```python
from build123d import *

# Parameters (mm, degrees)
BASE_DEPTH          = 3
SKETCH2_R           = 1.5
CUT_EXTRUDE1_DEPTH  = 37.373066959
CUT_EXTRUDE2_DEPTH  = 37.373066959
SKETCH6_R           = 3
CUT_EXTRUDE3_DEPTH  = 1.5
CHAMFER2_SIZE       = 0.5
BOSS_EXTRUDE1_START = -2.5
BOSS_EXTRUDE1_DEPTH = 2.5
CUT_EXTRUDE4_START  = -2.5
CUT_EXTRUDE4_DEPTH  = 2.5


# Read off the part's stored shape, not the designer's step: Cut-Extrude4
with BuildPart() as part:
    # Sketch1 → Base (new body)
    with BuildSketch(Plane.XY):
        with BuildLine():
            Line((11, -33), (-11, -33))
            ThreePointArc((-11, -33), (-13.828427125, -31.828427125), (-15, -29))
            Line((-15, -29), (-15, 29))
            ThreePointArc((-15, 29), (-13.828427125, 31.828427125), (-11, 33))
            Line((-11, 33), (11, 33))
            ThreePointArc((11, 33), (13.828427125, 31.828427125), (15, 29))
            Line((15, 29), (15, -29))
            ThreePointArc((15, -29), (13.828427125, -31.828427125), (11, -33))
        make_face()
    extrude(amount=BASE_DEPTH)

    # Sketch2 → Cut-Extrude1 (cut, through all)
    with BuildSketch(Plane.XY.offset(3)):
        with Locations((-11, 29)):
            Circle(SKETCH2_R)
        with Locations((-11, -29)):
            Circle(SKETCH2_R)
        with Locations((11, -29)):
            Circle(SKETCH2_R)
        with Locations((11, 29)):
            Circle(SKETCH2_R)
    extrude(amount=-CUT_EXTRUDE1_DEPTH, mode=Mode.SUBTRACT)

    # Sketch3 → Cut-Extrude2 (cut, through all)
    with BuildSketch(Plane.XY.offset(3)):
        with BuildLine():
            Line((6.5, 29), (6.5, 31))
            Line((6.5, 31), (-6.5, 31))
            Line((-6.5, 31), (-6.5, 29))
            ThreePointArc((-6.5, 29), (-7.818019485, 25.818019485), (-11, 24.5))
            Line((-11, 24.5), (-13, 24.5))
            Line((-13, 24.5), (-13, -24.5))
            Line((-13, -24.5), (-11, -24.5))
            ThreePointArc((-11, -24.5), (-7.818019485, -25.818019485), (-6.5, -29))
            Line((-6.5, -29), (-6.5, -31))
            Line((-6.5, -31), (6.5, -31))
            Line((6.5, -31), (6.5, -29))
            ThreePointArc((6.5, -29), (7.818019485, -25.818019485), (11, -24.5))
            Line((11, -24.5), (13, -24.5))
            Line((13, -24.5), (13, 24.5))
            Line((13, 24.5), (11, 24.5))
            ThreePointArc((11, 24.5), (7.818019485, 25.818019485), (6.5, 29))
        make_face()
    extrude(amount=-CUT_EXTRUDE2_DEPTH, mode=Mode.SUBTRACT)

    # Sketch6 → Cut-Extrude3 (cut)
    with BuildSketch(Plane.XY.offset(3)):
        with Locations((-11, -29)):
            Circle(SKETCH6_R)
        with Locations((11, -29)):
            Circle(SKETCH6_R)
        with Locations((11, 29)):
            Circle(SKETCH6_R)
        with Locations((-11, 29)):
            Circle(SKETCH6_R)
    extrude(amount=-CUT_EXTRUDE3_DEPTH, mode=Mode.SUBTRACT)

    # Chamfer2
    chamfer2_edges = [part.edges().sort_by_distance(p)[0] for p in [
        (7.818019485, 25.818019485, 3),
        (13, 0, 3),
        (7.818019485, -25.818019485, 3),
        (-7.818019485, -25.818019485, 3),
        (-13, 0, 3),
        (-7.818019485, 25.818019485, 3),
        (0, -33, 3),
        (-13.828427125, -31.828427125, 3),
        (-15, 0, 3),
        (-13.828427125, 31.828427125, 3),
        (0, 33, 3),
        (13.828427125, 31.828427125, 3),
        (15, 0, 3),
        (13.828427125, -31.828427125, 3),
        (-14, -29, 3),
        (-14, 29, 3),
        (8, 29, 3),
        (8, -29, 3),
        (0, -31, 3),
        (0, 31, 3),
        (12, 24.5, 3),
        (6.5, 30, 3),
        (-6.5, 30, 3),
        (-12, 24.5, 3),
        (-12, -24.5, 3),
        (-6.5, -30, 3),
        (6.5, -30, 3),
        (12, -24.5, 3),
    ]]
    chamfer(chamfer2_edges, length=CHAMFER2_SIZE - 0.0001)  # a hair under: the kernel refuses the full size

    # Sketch9 → Boss-Extrude1 (add)
    with BuildSketch(Plane(origin=(0, 0, 0), x_dir=(-1, 0, 0), z_dir=(0, 0, -1)).offset(BOSS_EXTRUDE1_START)):
        with BuildLine():
            ThreePointArc((-6.5, -29), (-7.818019485, -25.818019485), (-11, -24.5))
            Line((-11, -24.5), (-13, -24.5))
            Line((-13, -24.5), (-13, 24.5))
            Line((-13, 24.5), (-11, 24.5))
            ThreePointArc((-11, 24.5), (-7.818019485, 25.818019485), (-6.5, 29))
            Line((-6.5, 29), (-6.5, 31))
            Line((-6.5, 31), (6.5, 31))
            Line((6.5, 31), (6.5, 29))
            ThreePointArc((6.5, 29), (7.818019485, 25.818019485), (11, 24.5))
            Line((11, 24.5), (13, 24.5))
            Line((13, 24.5), (13, -24.5))
            Line((13, -24.5), (11, -24.5))
            ThreePointArc((11, -24.5), (7.818019485, -25.818019485), (6.5, -29))
            Line((6.5, -29), (6.5, -31))
            Line((6.5, -31), (-6.5, -31))
            Line((-6.5, -31), (-6.5, -29))
        make_face()
    extrude(amount=BOSS_EXTRUDE1_DEPTH)

    # Cut-Extrude4 outline → Cut-Extrude4 (cut)
    with BuildSketch(Plane(origin=(0, 0, 0), x_dir=(-1, 0, 0), z_dir=(0, 0, -1)).offset(CUT_EXTRUDE4_START)):
        with BuildLine():
            ThreePointArc((11.25, -6.45), (12.8, -4.9), (11.25, -3.35))
            Line((11.25, -3.35), (-11.25, -3.35))
            ThreePointArc((-11.25, -3.35), (-12.8, -4.9), (-11.25, -6.45))
            Line((-11.25, -6.45), (11.25, -6.45))
        make_face()
        with BuildLine():
            ThreePointArc((11.25, 18.05), (12.8, 19.6), (11.25, 21.15))
            Line((11.25, 21.15), (-11.25, 21.15))
            ThreePointArc((-11.25, 21.15), (-12.8, 19.6), (-11.25, 18.05))
            Line((-11.25, 18.05), (11.25, 18.05))
        make_face()
        with BuildLine():
            Line((-11, 24.5), (-12.8, 24.5))
            ThreePointArc((-12.8, 24.5), (-12.346015511, 23.403984489), (-11.25, 22.95))
            Line((-11.25, 22.95), (11.25, 22.95))
            ThreePointArc((11.25, 22.95), (12.346015511, 23.403984489), (12.8, 24.5))
            Line((12.8, 24.5), (11, 24.5))
            ThreePointArc((11, 24.5), (9.13251506, 24.905796781), (7.601838732, 26.05))
            Line((7.601838732, 26.05), (-7.601838732, 26.05))
            ThreePointArc((-7.601838732, 26.05), (-9.13251506, 24.905796781), (-11, 24.5))
        make_face()
        with BuildLine():
            ThreePointArc((-6.5, 29), (-6.537512687, 28.420166419), (-6.649425325, 27.85))
            Line((-6.649425325, 27.85), (6.649425325, 27.85))
            ThreePointArc((6.649425325, 27.85), (6.537512687, 28.420166419), (6.5, 29))
            Line((6.5, 29), (6.5, 30.95))
            Line((6.5, 30.95), (-6.5, 30.95))
            Line((-6.5, 30.95), (-6.5, 29))
        make_face()
        with BuildLine():
            Line((6.5, -30.95), (6.5, -29))
            ThreePointArc((6.5, -29), (6.537512687, -28.420166419), (6.649425325, -27.85))
            Line((6.649425325, -27.85), (-6.649425325, -27.85))
            ThreePointArc((-6.649425325, -27.85), (-6.537512687, -28.420166419), (-6.5, -29))
            Line((-6.5, -29), (-6.5, -30.95))
            Line((-6.5, -30.95), (6.5, -30.95))
        make_face()
        with BuildLine():
            Line((-11.25, -1.55), (11.25, -1.55))
            ThreePointArc((11.25, -1.55), (12.8, 0), (11.25, 1.55))
            Line((11.25, 1.55), (-11.25, 1.55))
            ThreePointArc((-11.25, 1.55), (-12.8, 0), (-11.25, -1.55))
        make_face()
        with BuildLine():
            ThreePointArc((11.25, -11.35), (12.8, -9.8), (11.25, -8.25))
            Line((11.25, -8.25), (-11.25, -8.25))
            ThreePointArc((-11.25, -8.25), (-12.8, -9.8), (-11.25, -11.35))
            Line((-11.25, -11.35), (11.25, -11.35))
        make_face()
        with BuildLine():
            ThreePointArc((11.25, -16.25), (12.8, -14.7), (11.25, -13.15))
            Line((11.25, -13.15), (-11.25, -13.15))
            ThreePointArc((-11.25, -13.15), (-12.8, -14.7), (-11.25, -16.25))
            Line((-11.25, -16.25), (11.25, -16.25))
        make_face()
        with BuildLine():
            ThreePointArc((11.25, -21.15), (12.8, -19.6), (11.25, -18.05))
            Line((11.25, -18.05), (-11.25, -18.05))
            ThreePointArc((-11.25, -18.05), (-12.8, -19.6), (-11.25, -21.15))
            Line((-11.25, -21.15), (11.25, -21.15))
        make_face()
        with BuildLine():
            ThreePointArc((12.8, -24.5), (12.346015511, -23.403984489), (11.25, -22.95))
            Line((11.25, -22.95), (-11.25, -22.95))
            ThreePointArc((-11.25, -22.95), (-12.346015511, -23.403984489), (-12.8, -24.5))
            Line((-12.8, -24.5), (-11, -24.5))
            ThreePointArc((-11, -24.5), (-9.13251506, -24.905796781), (-7.601838732, -26.05))
            Line((-7.601838732, -26.05), (7.601838732, -26.05))
            ThreePointArc((7.601838732, -26.05), (9.13251506, -24.905796781), (11, -24.5))
            Line((11, -24.5), (12.8, -24.5))
        make_face()
        with BuildLine():
            ThreePointArc((11.25, 3.35), (12.8, 4.9), (11.25, 6.45))
            Line((11.25, 6.45), (-11.25, 6.45))
            ThreePointArc((-11.25, 6.45), (-12.8, 4.9), (-11.25, 3.35))
            Line((-11.25, 3.35), (11.25, 3.35))
        make_face()
        with BuildLine():
            ThreePointArc((11.25, 8.25), (12.8, 9.8), (11.25, 11.35))
            Line((11.25, 11.35), (-11.25, 11.35))
            ThreePointArc((-11.25, 11.35), (-12.8, 9.8), (-11.25, 8.25))
            Line((-11.25, 8.25), (11.25, 8.25))
        make_face()
        with BuildLine():
            ThreePointArc((11.25, 13.15), (12.8, 14.7), (11.25, 16.25))
            Line((11.25, 16.25), (-11.25, 16.25))
            ThreePointArc((-11.25, 16.25), (-12.8, 14.7), (-11.25, 13.15))
            Line((-11.25, 13.15), (11.25, 13.15))
        make_face()
    extrude(amount=CUT_EXTRUDE4_DEPTH, mode=Mode.SUBTRACT)


solid = part.part
```
Verification items for the finished model (mm, model axes). A direction names the side the tool comes from. Coordinates: 2 decimals unless noted, no trailing zeros. Write each loop counter-clockwise with the first axis right and the second up, starting at its lowest first coordinate (ties: lowest second). Pieces come first, ordered by that corner, then holes. Notation, with made-up numbers: M 55,78 L 63,78 A36 ccw 63,116 Z; hole C 73,-36 d6. An arc over 180 degrees is marked long. Answer as a JSON object with one key per item and string values. Group by question number.
(1) Tool access check on faces 5 (the face through (12.8, -9.8, 1.3)), 6 (the face through (-9.7, -30.3, 1.5)). Record the directions out of +Z, -Z, +X, -X, +Y, -Y that give a thin tool (end or side, any length) a straight path to the whole face; none if there is none.
(2) Cross-section at A-A, the plane y = -4.9. Record the cut outline in (x, z).
(3) Material ranges on line 1 (X direction, y = -27, z = 2.05); line 2 (Z direction, x = -9, y = -2.5); line 3 (Y direction, x = 4.5, z = 2.85), recorded low to high.
(4) Gauge pin test, flat ends, axial feed: pin 1 (1.5 mm diameter, centred on x = 11, y = -19, fed in from +Z); pin 2 (4 mm diameter, centred on x = 5, y = 7.5, fed in from +Z); pin 3 (3.5 mm diameter, centred on x = 11, y = -29, fed in from +Z); pin 4 (1.6 mm diameter, centred on x = 12.5, z = 1.5, fed in from -Y). Record the tip position at first contact, or that the pin passes through.
(5) Cross-section at B-B, the plane x = 3.75. State how many separate pieces and enclosed holes the cut face has, and give its area (3 significant figures).
(6) Release check for a two-part mould opening along Y. For faces 1 (the face through (15, 0, 1)), 2 (the face through (0, -33, 1)), 3 (the face through (-6.5, 30, 1)), 4 (the face through (0, -1.55, 1)) record: +Y half, -Y half, draft (parallel to the pull), parting line (faces both ways), or undercut.
Reply:
{
 "1": {"face 5": "+Z, -Z", "face 6": "+Z"},
 "2": {"outline": "M -15,0 L -12.8,0 L -12.8,2.5 L -13,2.5 L -13.5,3 L -14.5,3 L -15,2.5 Z; M 12.8,0 L 15,0 L 15,2.5 L 14.5,3 L 13.5,3 L 13,2.5 L 12.8,2.5 Z"},
 "3": {"line 1": "-15 to -13.24, -8.76 to 8.76, 13.24 to 15", "line 2": "0 to 2.5", "line 3": "-32.65 to -31.35, 31.35 to 32.65"},
 "4": {"pin 1": "through", "pin 2": "z = 2.5", "pin 3": "z = 1.5", "pin 4": "y = -32.94"},
 "5": {"separate pieces": "14", "enclosed holes": "0", "area": "65.8 mm²"},
 "6": {"face 1": "draft", "face 2": "-Y half", "face 3": "undercut", "face 4": "undercut"}
}
